Read the model definition and answer for the solid it produces. Units are mm, in the model's axes. Coordinates: 2 decimals unless noted, no trailing zeros. Order: outer loops, then holes, each group sorted by start corner. A loop starts at its lowest first (then second) coordinate and runs counter-clockwise, first axis right, second up.
```python
from build123d import *

# Parameters (mm, degrees)
SKETCH1_W           = 152.4
SKETCH1_H           = 152.4
SKETCH1_R           = 1.2
BOSS_EXTRUDE1_DEPTH = 1.5748
SKETCH2_W           = 30
SKETCH2_H           = 50
CUT_EXTRUDE1_DEPTH  = 2.5748


with BuildPart() as part:
    # Sketch1 → Boss-Extrude1 (new body)
    with BuildSketch(Plane(origin=(0, 0, 0), x_dir=(1, 0, 0), z_dir=(0, 1, 0))):
        Rectangle(SKETCH1_W, SKETCH1_H)
        with Locations((-51.7, 73.8)):
            Circle(SKETCH1_R, mode=Mode.SUBTRACT)
        with Locations((51.7, 73.8)):
            Circle(SKETCH1_R, mode=Mode.SUBTRACT)
        with Locations((73.8, 51.7)):
            Circle(SKETCH1_R, mode=Mode.SUBTRACT)
        with Locations((73.8, -51.7)):
            Circle(SKETCH1_R, mode=Mode.SUBTRACT)
        with Locations((-73.8, -51.7)):
            Circle(SKETCH1_R, mode=Mode.SUBTRACT)
        with Locations((-73.8, 51.7)):
            Circle(SKETCH1_R, mode=Mode.SUBTRACT)
        with Locations((-51.7, -73.8)):
            Circle(SKETCH1_R, mode=Mode.SUBTRACT)
        with Locations((51.7, -73.8)):
            Circle(SKETCH1_R, mode=Mode.SUBTRACT)
    extrude(amount=BOSS_EXTRUDE1_DEPTH)

    # Sketch2 → Cut-Extrude1 (cut, through all)
    with BuildSketch(Plane(origin=(0, 1.5748, 0), x_dir=(1, 0, 0), z_dir=(0, 1, 0))):
        with Locations((-61.2, 51.2)):
            Rectangle(SKETCH2_W, SKETCH2_H)
    extrude(amount=-CUT_EXTRUDE1_DEPTH, mode=Mode.SUBTRACT)


solid = part.part
```
1) A flat-ended cylindrical pin translates along its axis: pin 1 Ø4 at (x, z) = (-51.7, 73.8) entering from -Y. Find the tip coordinate at first contact, or state that the pin passes through.
A:
pin 1: stops at y = 0
2) A cutting plane is placed at B-B, the plane z = -33.5. Determine the outline of the cut face in (x, y), and give its area (3 significant figures).
A:
outline: (-46.2, 0) - (76.2, 0) - (76.2, 1.57) - (-46.2, 1.57) - close
area: 193 mm2
3) Straight lines are drawn through the part: line 1 (X direction, y = 0.75, z = 73.8); line 2 (X direction, y = 0.7, z = 51.7). For each, find the intervals that lie inside material, in ascending order.
A:
line 1: x = -76.2 to -52.9, -50.5 to 50.5, 52.9 to 76.2
line 2: x = -76.2 to -75, -72.6 to 72.6, 75 to 76.2
4) A cutting plane is placed at A-A, the plane y = 0.65. Determine the outline of the cut face in (x, z), and give its area (3 significant figures).
A:
outline: (-76.2, -26.2) - (-46.2, -26.2) - (-46.2, -76.2) - (76.2, -76.2) - (76.2, 76.2) - (-76.2, 76.2) - close; hole circle Ø2.4 at (-73.8, 51.7); hole circle Ø2.4 at (-51.7, 73.8); hole circle Ø2.4 at (51.7, -73.8); hole circle Ø2.4 at (51.7, 73.8); hole circle Ø2.4 at (73.8, -51.7); hole circle Ø2.4 at (73.8, 51.7)
area: 21,700 mm2
